Part print with two shaded views. Sizes in mm from the minimum x, y, z corner. A direction names the side the tool comes from. Round coordinates to 2 decimals unless told otherwise and drop trailing zeros. Loops run counter-clockwise (first coordinate to the right, second up) from the corner with the lowest first, then second, coordinate; pieces in that order, holes last. Notation, with made-up numbers: (-22, 59) -> (23, 59) arc R27 ccw to (23, 88) -> close; hole circle Ø8 at (59.5, 55). An arc over 180 degrees is marked (long way). Use a Markdown table: item, result. Add a question column.
Item 1: Cut at A-A, the plane y = 36.5. List the corners of the cut face in (x, z), plus the area to 3 significant figures.
Item 2: Cut at B-B, the plane x = 30. List the corners of the cut face in (y, z).
Item 3: Cut at C-C, the plane z = 19.5. List the corners of the cut face in (x, y).
Item 4: Flat gauge pins, fed straight in: pin 1 (10.5 mm diameter, centred on x = 26, z = 77.5, fed in from +Y); pin 2 (10.5 mm diameter, centred on x = 16.5, z = 40, fed in from +Y); pin 3 (8 mm diameter, centred on x = 10, y = 29, fed in from +Z). Where does each tip first touch, or does it go through?
Item 5: Which spindle directions (+Z, -Z, +X, -X, +Y, -Y) get a long thin tool onto all of the face, cutting with end or side? Do the marked faces 4, 5, 6 and 7. Say none if no direction does.
Item 6: Probe line 1 (X direction, y = 14, z = 58.5); line 2 (Z direction, x = 35.5, y = 6); line 3 (X direction, y = 36.5, z = 23.75). List the from-to ranges inside material, lowest first. Write a range as [from, to].
Item 7: Cut at D-D, the plane x = 51. List the corners of the cut face in (y, z), plus the area to 3 significant figures.
Item 8: Two-plate mould, pull along X, no slides. Class the marked faces 1, 2 and 3: pulls with the +X half, pulls with the -X half, needs draft (parallel to the pull), parting line crosses it, or undercut.
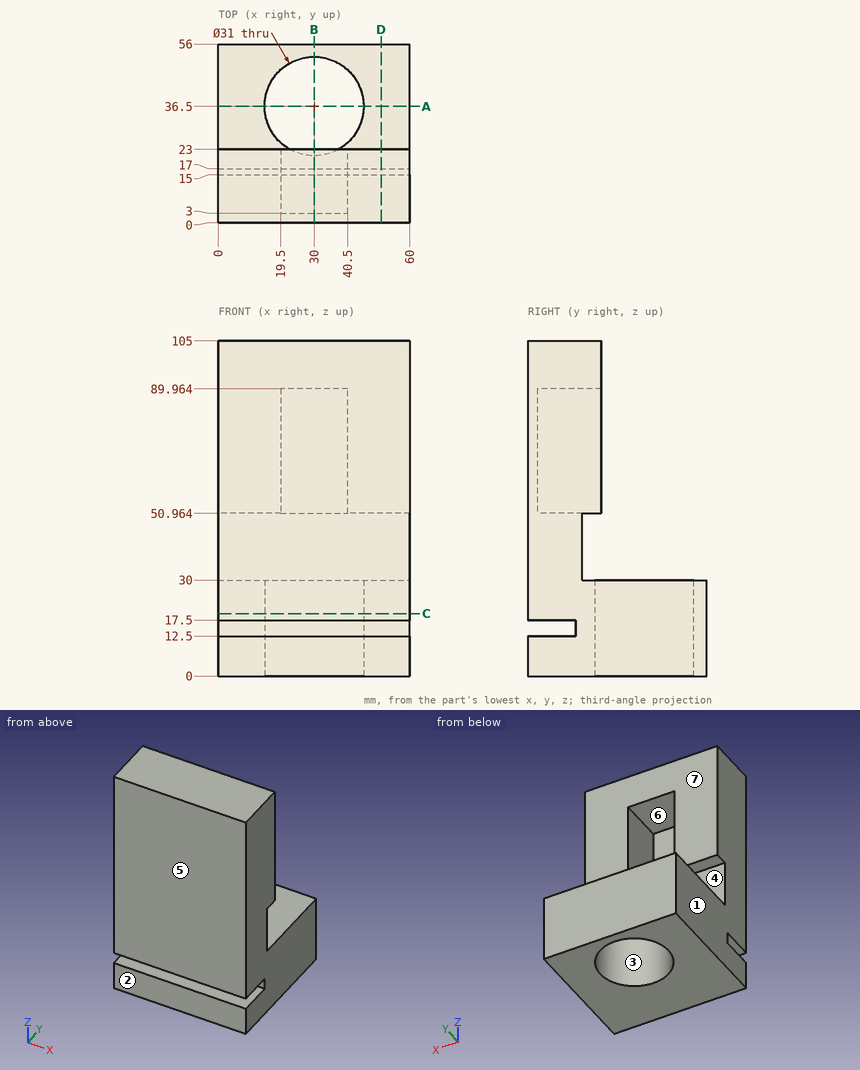
A:
| question | item | result |
|---|---|---|
| 1 | outline | (0, 0) -> (14.5, 0) -> (14.5, 30) -> (0, 30) -> close; (45.5, 0) -> (60, 0) -> (60, 30) -> (45.5, 30) -> close |
| 1 | area | 870 mm^2 |
| 2 | outline | (0, 0) -> (21, 0) -> (21, 30) -> (17, 30) -> (17, 50.96) -> (3, 50.96) -> (3, 89.96) -> (23, 89.96) -> (23, 105) -> (0, 105) -> (0, 17.5) -> (15, 17.5) -> (15, 12.5) -> (0, 12.5) -> close; (52, 0) -> (56, 0) -> (56, 30) -> (52, 30) -> close |
| 3 | outline | (0, 0) -> (60, 0) -> (60, 56) -> (0, 56) -> close; hole circle Ø31 at (30, 36.5) |
| 4 | pin 1 | stops at y = 3 |
| 4 | pin 2 | stops at y = 17 |
| 4 | pin 3 | stops at z = 30 |
| 5 | face 4 | +X, -X, +Y |
| 5 | face 5 | +Z, -Z, +X, -X, -Y |
| 5 | face 6 | +Y |
| 5 | face 7 | +Z, +X, -X, +Y |
| 6 | line 1 | x = [0, 19.5], [40.5, 60] |
| 6 | line 2 | z = [0, 12.5], [17.5, 50.96], [89.96, 105] |
| 6 | line 3 | x = [0, 14.5], [45.5, 60] |
| 7 | outline | (0, 0) -> (56, 0) -> (56, 30) -> (17, 30) -> (17, 50.96) -> (23, 50.96) -> (23, 105) -> (0, 105) -> (0, 17.5) -> (15, 17.5) -> (15, 12.5) -> (0, 12.5) -> close |
| 7 | area | 3,200 mm^2 |
| 8 | face 1 | pulls with the -X half |
| 8 | face 2 | needs draft |
| 8 | face 3 | undercut |
